```python
from build123d import *

# Parameters (mm, degrees)
BOSS_EXTRU_1_DEPTH      = 173
D_GAGEMENT_M31_D        = 3.2
D_GAGEMENT_M31_DEPTH    = 5
D_GAGEMENT_M31_TIP      = 0.96137699
ENL_V_MAT_EXTRU_1_DEPTH = 56


with BuildPart() as part:
    # Esquisse1 → Boss.-Extru.1 (new body)
    with BuildSketch(Plane.XY):
        with BuildLine():
            Line((-81.597369332, 0), (-76.402630668, 0))
            ThreePointArc((-76.402630668, 0), (-69.473365186, 2.789918178), (-66.41051645, 9.602944025))
            Line((-66.41051645, 9.602944025), (-64.996057109, 45.198527987))
            ThreePointArc((-64.996057109, 45.198527987), (-63.464632741, 48.605040911), (-60, 50))
            Line((-60, 50), (60, 50))
            ThreePointArc((60, 50), (63.464632741, 48.605040911), (64.996057109, 45.198527987))
            Line((64.996057109, 45.198527987), (66.41051645, 9.602944025))
            ThreePointArc((66.41051645, 9.602944025), (69.473365186, 2.789918178), (76.402630668, 0))
            Line((76.402630668, 0), (81.597369332, 0))
            Line((81.597369332, 0), (81.597369332, 5))
            Line((81.597369332, 5), (76.402630668, 5))
            ThreePointArc((76.402630668, 5), (72.937997927, 6.394959089), (71.406573559, 9.801472013))
            Line((71.406573559, 9.801472013), (69.992114218, 45.397055975))
            ThreePointArc((69.992114218, 45.397055975), (66.929265482, 52.210081822), (60, 55))
            Line((60, 55), (-60, 55))
            ThreePointArc((-60, 55), (-66.929265482, 52.210081822), (-69.992114218, 45.397055975))
            Line((-69.992114218, 45.397055975), (-71.406573559, 9.801472013))
            ThreePointArc((-71.406573559, 9.801472013), (-72.937997927, 6.394959089), (-76.402630668, 5))
            Line((-76.402630668, 5), (-81.597369332, 5))
            Line((-81.597369332, 5), (-81.597369332, 0))
        make_face()
    extrude(amount=BOSS_EXTRU_1_DEPTH)

    # Dégagement M31
    with Locations(Plane(origin=(0, 5, 0), x_dir=(1, 0, 0), z_dir=(0, 1, 0))):
        with Locations((-79, -170), (-79, -3), (79, -170), (79, -3)):
            Hole(D_GAGEMENT_M31_D / 2, depth=D_GAGEMENT_M31_DEPTH)
            with Locations((0, 0, -(D_GAGEMENT_M31_DEPTH + D_GAGEMENT_M31_TIP / 2))):  # 118° drill point
                Cone(0, D_GAGEMENT_M31_D / 2, D_GAGEMENT_M31_TIP, mode=Mode.SUBTRACT)

    # Esquisse4 → Enlèv. mat.-Extru.1 (cut, through all)
    with BuildSketch(Plane(origin=(0, 55, 0), x_dir=(1, 0, 0), z_dir=(0, 1, 0))):
        with BuildLine():
            ThreePointArc((-20.093103017, -131.5), (-41.306306452, -122.713203436), (-50.093103017, -101.5))
            Line((-50.093103017, -101.5), (-50.093103017, -71.5))
            ThreePointArc((-50.093103017, -71.5), (-41.306306452, -50.286796564), (-20.093103017, -41.5))
            Line((-20.093103017, -41.5), (20.093103017, -41.5))
            ThreePointArc((20.093103017, -41.5), (41.306306452, -50.286796564), (50.093103017, -71.5))
            Line((50.093103017, -71.5), (50.093103017, -101.5))
            ThreePointArc((50.093103017, -101.5), (41.306306452, -122.713203436), (20.093103017, -131.5))
            Line((20.093103017, -131.5), (-20.093103017, -131.5))
        make_face()
        with BuildLine():
            ThreePointArc((81.366251775, -168.928935118), (81.538932575, -169.4521416), (81.597369332, -170))
            Line((81.597369332, -170), (81.597369332, -3))
            ThreePointArc((81.597369332, -3), (81.538932575, -3.5478584), (81.366251775, -4.071064882))
            Line((81.366251775, -4.071064882), (62.762544981, -45.171333393))
            ThreePointArc((62.762544981, -45.171333393), (60.768056204, -51.214445653), (60.093103017, -57.542291215))
            Line((60.093103017, -57.542291215), (60.093103017, -115.457708785))
            ThreePointArc((60.093103017, -115.457708785), (60.768056204, -121.785554347), (62.762544981, -127.828666607))
            Line((62.762544981, -127.828666607), (81.366251775, -168.928935118))
        make_face()
        with BuildLine():
            Line((60, -0.402630668), (-60, -0.402630668))
            Line((-60, -0.402630668), (-60, -17.351236736))
            Line((-60, -17.351236736), (-53.668539182, -23.323392752))
            ThreePointArc((-53.668539182, -23.323392752), (-44.158310479, -29.381013096), (-33.083604671, -31.5))
            Line((-33.083604671, -31.5), (33.083604671, -31.5))
            ThreePointArc((33.083604671, -31.5), (44.158310479, -29.381013096), (53.668539182, -23.323392752))
            Line((53.668539182, -23.323392752), (60, -17.351236736))
            Line((60, -17.351236736), (60, -0.402630668))
        make_face()
        with BuildLine():
            Line((-60, -0.402630668), (-79, -0.402630668))
            ThreePointArc((-79, -0.402630668), (-78.041163293, -0.586090388), (-77.217777414, -1.110552965))
            Line((-77.217777414, -1.110552965), (-60, -17.351236736))
            Line((-60, -17.351236736), (-60, -0.402630668))
        make_face()
        with BuildLine():
            Line((79, -0.402630668), (60, -0.402630668))
            Line((60, -0.402630668), (60, -17.351236736))
            Line((60, -17.351236736), (77.217777414, -1.110552965))
            ThreePointArc((77.217777414, -1.110552965), (78.041163293, -0.586090388), (79, -0.402630668))
        make_face()
        with BuildLine():
            ThreePointArc((-81.597369332, -170), (-81.538932575, -169.4521416), (-81.366251775, -168.928935118))
            Line((-81.366251775, -168.928935118), (-62.762544981, -127.828666607))
            ThreePointArc((-62.762544981, -127.828666607), (-60.768056204, -121.785554347), (-60.093103017, -115.457708785))
            Line((-60.093103017, -115.457708785), (-60.093103017, -57.542291215))
            ThreePointArc((-60.093103017, -57.542291215), (-60.768056204, -51.214445653), (-62.762544981, -45.171333393))
            Line((-62.762544981, -45.171333393), (-81.366251775, -4.071064882))
            ThreePointArc((-81.366251775, -4.071064882), (-81.538932575, -3.5478584), (-81.597369332, -3))
            Line((-81.597369332, -3), (-81.597369332, -170))
        make_face()
        with BuildLine():
            Line((-60, -155.648763264), (-60, -172.597369332))
            Line((-60, -172.597369332), (60, -172.597369332))
            Line((60, -172.597369332), (60, -155.648763264))
            Line((60, -155.648763264), (53.668539182, -149.676607248))
            ThreePointArc((53.668539182, -149.676607248), (44.158310479, -143.618986904), (33.083604671, -141.5))
            Line((33.083604671, -141.5), (-33.083604671, -141.5))
            ThreePointArc((-33.083604671, -141.5), (-44.158310479, -143.618986904), (-53.668539182, -149.676607248))
            Line((-53.668539182, -149.676607248), (-60, -155.648763264))
        make_face()
        with BuildLine():
            Line((60, -155.648763264), (60, -172.597369332))
            Line((60, -172.597369332), (79, -172.597369332))
            ThreePointArc((79, -172.597369332), (78.041163293, -172.413909612), (77.217777414, -171.889447035))
            Line((77.217777414, -171.889447035), (60, -155.648763264))
        make_face()
        with BuildLine():
            ThreePointArc((-77.217777414, -171.889447035), (-78.041163293, -172.413909612), (-79, -172.597369332))
            Line((-79, -172.597369332), (-60, -172.597369332))
            Line((-60, -172.597369332), (-60, -155.648763264))
            Line((-60, -155.648763264), (-77.217777414, -171.889447035))
        make_face()
    extrude(amount=-ENL_V_MAT_EXTRU_1_DEPTH, mode=Mode.SUBTRACT)


solid = part.part
```
Source: CAD feature listing. Evaluate the final solid. Frame: model axes, mm. A direction names the side the tool comes from. Give positions to 0.01 mm unless a question says otherwise; leave off trailing zeros. Loops run counter-clockwise (first coordinate to the right, second up) from the corner with the lowest first, then second, coordinate; pieces in that order, holes last. Notation, with made-up numbers: (-5.5, 5.5) -> (44.5, 5.5) arc R17 ccw to (44.5, 35.5) -> close; hole circle Ø8 at (65.25, 6). An arc over 180 degrees is marked (long way). Put each result on its own line as item: value. Start each with the question number.
1) Material intervals for probe 1 along X at (y, z) = (1.2, 170); probe 2 along X at (y, z) = (45.5, 138.5); probe 3 along X at (y, z) = (11.5, 148), sorted ascending.
2) Contact query for flat-ended pins moving along their axis: P1, Ø4, axis at y = 53, z = 89.5, coming from the +X side; P2, Ø1.6, axis at x = 78, z = 5.5, coming from the +Y side; P3, Ø1, axis at x = -55.5, z = 69.5, coming from the -Y side. Output: stop coordinate, or through.
3) Cut plane C-C (y = 7.5). State how many separate pieces and enclosed holes the cut face has, then the cut area to 3 significant figures.
4) Draft query along X for faces 5 (the face through (-41.538, 52.535, 50.521)), 6 (the face through (-69.352, 25.41, 142.386)), 7 (the face through (67.006, 52.135, 0.198)). Return one class per face: released by +X, released by -X, zero draft, split by the parting line, or undercut.
5) Reachability of faces 1 (the face through (78, 5, 167)), 2 (the face through (-78, 5, 167)), 3 (the face through (0, 53, 31.5)), 4 (the face through (65.693, 27.65, 147.027)) from +Z, -Z, +X, -X, +Y, -Y: full face, straight path, thin tool, end or side. Return the list, or none.
6) Cut plane B-B (x = 14.5). Return loops of the section in (y, z).
7) Cut plane A-A (z = 90.5). Return loops of the section in (x, y), then the cut area to 3 significant figures.
Results are:
1. probe 1: x = -81.6 to -80.6, -77.4 to -75.21, 75.21 to 77.4, 80.6 to 81.6
1. probe 2: x = -67.59 to -64.97, 64.97 to 67.59
1. probe 3: x = -71.34 to -66.34, 66.34 to 71.34
2. P1: stops at x = 60.09
2. P2: stops at y = 5
2. P3: stops at y = 50
3. separate pieces: 8
3. enclosed holes: 0
3. area: 480 mm2
4. face 5: undercut
4. face 6: released by -X
4. face 7: released by +X
5. face 1: +Z, -Z, +X, +Y
5. face 2: +Z, -Z, -X, +Y
5. face 3: +Y, -Y
5. face 4: +Z, -Z, -Y
6. outline: (50, 0) -> (55, 0) -> (55, 0.4) -> (50, 0.4) -> close; (50, 31.5) -> (55, 31.5) -> (55, 41.5) -> (50, 41.5) -> close; (50, 131.5) -> (55, 131.5) -> (55, 141.5) -> (50, 141.5) -> close; (50, 172.6) -> (55, 172.6) -> (55, 173) -> (50, 173) -> close
7. outline: (-60.09, 50) arc R5 cw to (-60, 50) -> (-50.09, 50) -> (-50.09, 55) -> (-60, 55) arc R10 ccw to (-60.09, 55) -> close; (50.09, 50) -> (60, 50) arc R5 cw to (60.09, 50) -> (60.09, 55) arc R10 ccw to (60, 55) -> (50.09, 55) -> close
7. area: 100 mm2
